Autodesk Inventor part; units mm, degrees
ref_plane "YZ Plane" through (0, 0, 0) normal (1, 0, 0) x (0, 1, 0)
ref_plane "XZ Plane" through (0, 0, 0) normal (0, 1, 0) x (-1, 0, 0)
ref_plane "XY Plane" through (0, 0, 0) normal (0, 0, 1) x (1, 0, 0)
sketch "Sketch1" plane through (0, 0, 0) normal (0, 0, 1) x (1, 0, 0)
  line L0 (134, 62) -> (131, 62)
  line L1 (131, 30) -> (134, 30)
  line L2 (134, 20) -> (134, 30)
  line L3 (134, 62) -> (134, 72)
  line L4 (3, 87) -> (3, 72)
  line L5 (3, 72) -> (0, 72)
  line L6 (0, 20) -> (3, 20)
  line L7 (3, 20) -> (3, 5)
  line L8 (0, 72) -> (0, 20)
  line L9 (131, 52) -> (121, 52)
  line L10 (119, 50) -> (119, 42)
  line L11 (121, 40) -> (131, 40)
  line L12 (131, 62) -> (131, 52)
  line L13 (131, 40) -> (131, 30)
  line L14 (106, 61.5) -> (116, 61.5)
  line L15 (116, 61.5) -> (116, 58.5)
  line L16 (116, 58.5) -> (106, 58.5)
  line L17 (106, 58.5) -> (106, 61.5)
  line L18 (106, 33.5) -> (116, 33.5)
  line L19 (116, 33.5) -> (116, 30.5)
  line L20 (116, 30.5) -> (106, 30.5)
  line L21 (106, 30.5) -> (106, 33.5)
  line L22 (88, 81) -> (91, 81)
  line L23 (91, 81) -> (91, 71)
  line L24 (91, 71) -> (88, 71)
  line L25 (88, 71) -> (88, 81)
  line L26 (88, 21) -> (91, 21)
  line L27 (91, 21) -> (91, 11)
  line L28 (91, 11) -> (88, 11)
  line L29 (88, 11) -> (88, 21)
  line L30 (134, 20) -> (127, 20)
  line L31 (125, 2) -> (125, 18)
  line L32 (134, 72) -> (127, 72)
  line L33 (125, 90) -> (125, 74)
  line L34 (49, 90) -> (49, 89)
  line L35 (51, 87) -> (77, 87)
  line L36 (79, 89) -> (79, 90)
  line L37 (123, 92) -> (81, 92)
  line L38 (49, 2) -> (49, 3)
  line L39 (51, 5) -> (77, 5)
  line L40 (79, 3) -> (79, 2)
  line L41 (81, 0) -> (123, 0)
  arc A0 (49, 90) -> (47, 92) centre (47, 90) ccw
  arc A1 (49, 89) -> (51, 87) centre (51, 89) ccw
  arc A2 (77, 87) -> (79, 89) centre (77, 89) ccw
  arc A3 (81, 92) -> (79, 90) centre (81, 90) ccw
  arc A4 (125, 74) -> (127, 72) centre (127, 74) ccw
  arc A5 (121, 52) -> (119, 50) centre (121, 50) ccw
  arc A6 (119, 42) -> (121, 40) centre (121, 42) ccw
  arc A7 (127, 20) -> (125, 18) centre (127, 18) ccw
  arc A8 (79, 2) -> (81, 0) centre (81, 2) ccw
  arc A9 (79, 3) -> (77, 5) centre (77, 3) ccw
  arc A10 (51, 5) -> (49, 3) centre (51, 3) ccw
  arc A11 (47, 0) -> (49, 2) centre (47, 2) ccw
  arc A12 (123, 0) -> (125, 2) centre (123, 2) ccw
  arc A13 (125, 90) -> (123, 92) centre (123, 90) ccw
  line L42 (3, 5) -> (13, 5)
  line L43 (13, 5) -> (13, 2)
  line L44 (15, 0) -> (47, 0)
  line L45 (3, 87) -> (13, 87)
  line L46 (13, 87) -> (13, 90)
  line L47 (47, 92) -> (15, 92)
  line L48 (26, 52) -> (36, 52)
  line L49 (37, 51) -> (37, 41)
  line L50 (36, 40) -> (26, 40)
  line L51 (25, 41) -> (25, 51)
  arc A14 (25, 41) -> (26, 40) centre (26, 41) ccw
  arc A15 (26, 52) -> (25, 51) centre (26, 51) ccw
  arc A16 (37, 51) -> (36, 52) centre (36, 51) ccw
  arc A17 (36, 40) -> (37, 41) centre (36, 41) ccw
  arc A18 (13, 2) -> (15, 0) centre (15, 2) ccw
  arc A19 (15, 92) -> (13, 90) centre (15, 90) ccw
  point P0 (0, 0)
  point P1 (125, 0)
  point P2 (125, 92)
  point P3 (119, 52)
  point P4 (119, 40)
  point P5 (125, 20)
  point P6 (125, 72)
  point P7 (49, 87)
  point P8 (79, 87)
  point P9 (79, 92)
  point P10 (49, 0)
  point P11 (49, 5)
  point P12 (79, 5)
  point P13 (79, 0)
  point P14 (13, 0)
  point P15 (13, 92)
  point P16 (25, 52)
  point P17 (37, 40)
  point P18 (37, 52)
  dimension "d6" = 52
  dimension "d8" = 10
  dimension "d12" = 10
  dimension "d14" = 3
  dimension "d15" = 3
  dimension "d19" = 12
  dimension "d20" = 12
  dimension "d22" = 10
  dimension "d24" = 10
  dimension "d26" = 10
  dimension "d27" = 10
  dimension "d28" = 3
  dimension "d29" = 3
  dimension "d30" = 25
  dimension "d32" = 15
  dimension "d33" = 3
  dimension "d34" = 10
  dimension "d35" = 10
  dimension "d36" = 3
  dimension "d46" = 40
  dimension "d47" = 20
  dimension "d48" = 9
  dimension "d51" = 3
  dimension "d67" = 46
  dimension "d69" = 30
  dimension "d70" = 30
  dimension "d74" = 46
  dimension "d76" = 122
  dimension "d77" = 2
  dimension "d78" = 2
  dimension "d79" = 3
  dimension "d80" = 128
  dimension "d81" = 40
  dimension "d90" = 12
  dimension "d91" = 12
  dimension "d92" = 25
  dimension "d95" = 40
  dimension "d96" = 1
  dimension "d99" = 9
  dimension "d102" = 82
  dimension "d103" = 5
  dimension "d104" = 5
  dimension "d105" = 2
extrude "Extrusion6" add sketch "Sketch1" along normal blind 3
properties part number "OpenROV_Dev_EChassis_Main_Plate"
Design review of the part built by this model. Coordinates are the model's own, in mm. A direction names the side the tool comes from. Coordinates: 2 decimals unless noted, no trailing zeros. Loops run counter-clockwise (first coordinate to the right, second up) from the corner with the lowest first, then second, coordinate; pieces in that order, holes last.
Q1. For pin 1 (0.9 mm diameter, centred on x = 60, z = 1, fed in from -Y); pin 2 (1 mm diameter, centred on y = 10.5, z = 1, fed in from -X); pin 3 (1.5 mm diameter, centred on y = 3.5, z = 1, fed in from -X), all flat-tipped, find the tip position at first contact; note any pin that passes through.
Reported:
pin 1: stops at y = 5
pin 2: stops at x = 3
pin 3: stops at x = 13
Q2. We need section B-B on z = 1.05. State how many separate pieces and enclosed holes the cut face has, and give its area (3 significant figures).
Reported:
separate pieces: 1
enclosed holes: 5
area: 10,900 mm2
Q3. Tool access review of faces 1 (the face through (132, 30, 1)), 2 (the face through (89, 81, 1)), 3 (the face through (13, 88, 1)), 4 (the face through (125, 10, 1)): name each direction out of +Z, -Z, +X, -X, +Y, -Y from which nothing blocks a thin tool from reaching the whole face with its end or side.
Reported:
face 1: +Z, -Z, +X
face 2: +Z, -Z
face 3: +Z, -Z, -X, +Y
face 4: +Z, -Z, +X, -Y
Q4. The part is to be moulded in two halves that separate along X. For faces 5 (the face through (131, 72, 1)), 6 (the face through (90, 11, 1)), 7 (the face through (0, 46, 1)), 8 (the face through (131, 57, 1)), say which applies: +X half, -X half, draft (parallel to the pull), parting line (faces both ways), or undercut.
Reported:
face 5: draft
face 6: undercut
face 7: -X half
face 8: +X half
Q5. We need section A-A on y = 48.5. State the section outline as (x, z) points.
Reported:
outline: (0, 0) - (25, 0) - (25, 3) - (0, 3) - close; (37, 0) - (119, 0) - (119, 3) - (37, 3) - close
Q6. We need section C-C on x = 8.5. State the section outline as (y, z) points.
Reported:
outline: (5, 0) - (87, 0) - (87, 3) - (5, 3) - close
Q7. To check wall thickness, follow line 1 (X direction, y = 76.5, z = 0.3); line 2 (X direction, y = 47.5, z = 0.8); line 3 (Y direction, x = 55, z = 0.8). State the ranges of each line that lie inside material, in increasing order.
Reported:
line 1: x = 3 to 88, 91 to 125
line 2: x = 0 to 25, 37 to 119
line 3: y = 5 to 87
